Verification items for the finished model (mm, model axes). A direction names the side the tool comes from. Coordinates: 2 decimals unless noted, no trailing zeros. Write each loop counter-clockwise with the first axis right and the second up, starting at its lowest first coordinate (ties: lowest second). Pieces come first, ordered by that corner, then holes. Notation, with made-up numbers: (54.5, -33) - (60.5, -33) arc R34 ccw to (60.5, 1) - close; hole circle Ø4 at (48.25, -30.5). An arc over 180 degrees is marked (long way). Use CSV: the item, a comma, the result in double quotes. Start each with the question number.
```python
from build123d import *

# Parameters (mm, degrees)
F0_R     = 3
F0_R_2   = 2.5
F1_DEPTH = 25


with BuildPart() as f1:
    # F0 (on Top) → F1 (new body)
    with BuildSketch(Plane.XY):
        with BuildLine():
            ThreePointArc((-14.5, 15), (-14.853553, 14.853553), (-15, 14.5))
            Line((-15, 14.5), (-15, 3.15))
            Line((-15, 3.15), (-12.5, 3.15))
            Line((-12.5, 3.15), (-12.5, 5.5))
            Line((-12.5, 5.5), (-6.90098, 5.5))
            ThreePointArc((-6.90098, 5.5), (-5.126404, 3.000613), (-4.5, 0))
            ThreePointArc((-4.5, 0), (-5.126404, -3.000613), (-6.90098, -5.5))
            Line((-6.90098, -5.5), (-12.5, -5.5))
            Line((-12.5, -5.5), (-12.5, -3.15))
            Line((-12.5, -3.15), (-15, -3.15))
            Line((-15, -3.15), (-15, -14.5))
            ThreePointArc((-15, -14.5), (-14.853553, -14.853553), (-14.5, -15))
            Line((-14.5, -15), (-3.15, -15))
            Line((-3.15, -15), (-3.15, -12.5))
            Line((-3.15, -12.5), (-5.5, -12.5))
            Line((-5.5, -12.5), (-5.5, -6.90098))
            ThreePointArc((-5.5, -6.90098), (-3.000613, -5.126404), (0, -4.5))
            ThreePointArc((0, -4.5), (3.000613, -5.126404), (5.5, -6.90098))
            Line((5.5, -6.90098), (5.5, -12.5))
            Line((5.5, -12.5), (3.15, -12.5))
            Line((3.15, -12.5), (3.15, -15))
            Line((3.15, -15), (14.5, -15))
            ThreePointArc((14.5, -15), (14.853553, -14.853553), (15, -14.5))
            Line((15, -14.5), (15, -3.15))
            Line((15, -3.15), (12.5, -3.15))
            Line((12.5, -3.15), (12.5, -5.5))
            Line((12.5, -5.5), (6.90098, -5.5))
            ThreePointArc((6.90098, -5.5), (5.126404, -3.000613), (4.5, 0))
            ThreePointArc((4.5, 0), (5.126404, 3.000613), (6.90098, 5.5))
            Line((6.90098, 5.5), (12.5, 5.5))
            Line((12.5, 5.5), (12.5, 3.15))
            Line((12.5, 3.15), (15, 3.15))
            Line((15, 3.15), (15, 14.5))
            ThreePointArc((15, 14.5), (14.853553, 14.853553), (14.5, 15))
            Line((14.5, 15), (3.15, 15))
            Line((3.15, 15), (3.15, 12.5))
            Line((3.15, 12.5), (5.5, 12.5))
            Line((5.5, 12.5), (5.5, 6.90098))
            ThreePointArc((5.5, 6.90098), (3.000613, 5.126404), (0, 4.5))
            ThreePointArc((0, 4.5), (-3.000613, 5.126404), (-5.5, 6.90098))
            Line((-5.5, 6.90098), (-5.5, 12.5))
            Line((-5.5, 12.5), (-3.15, 12.5))
            Line((-3.15, 12.5), (-3.15, 15))
            Line((-3.15, 15), (-14.5, 15))
        make_face()
        with Locations((-10, -10)):
            Circle(F0_R, mode=Mode.SUBTRACT)
        with Locations((10, -10)):
            Circle(F0_R, mode=Mode.SUBTRACT)
        Circle(F0_R_2, mode=Mode.SUBTRACT)
        with Locations((-10, 10)):
            Circle(F0_R, mode=Mode.SUBTRACT)
        with Locations((10, 10)):
            Circle(F0_R, mode=Mode.SUBTRACT)
    extrude(amount=F1_DEPTH)


solid = f1.part
```
Q1. Gauge pin test, flat end, axial feed: pin 1 (3 mm diameter, centred on x = 0, z = 11, fed in from -Y). Record the tip position at first contact, or that the pin passes through.
Q2. Cross-section at D-D (y = 0.5). Record the cut outline in (x, z), plus the area to 3 significant figures.
Q3. Cross-section at A-A (y = -10). Record the cut outline in (x, z), plus the area to 3 significant figures.
Q4. Scan lines: line 1 along Y through (x, z) = (10, 13.25); line 2 along Y through (x, z) = (-11.5, 5); line 3 along X through (y, z) = (-8, 5.25). Record each from-to range of solid material in increasing order. Write a range as from..to.
Q5. Tool access check on faces 1 (the flat face through (14, 3.15, 12)), 2 (the flat face through (4, -12.5, 12)). Record the directions out of +Z, -Z, +X, -X, +Y, -Y that give a thin tool (end or side, any length) a straight path to the whole face; none if there is none.
Q6. Cross-section at C-C (x = 1.75). Record the cut outline in (y, z).
Q7. Release check for a two-part mould opening along Y. For faces 3 (the flat face through (15, 9, 12)), 4 (the flat face through (-9, -15, 12)), 5 (the flat face through (10, -5.5, 12)), 6 (the flat face through (9, 15, 12)) record: released by +Y, released by -Y, zero draft, split by the parting line, or undercut.
Reply:
1,pin 1,"y = -4.65"
2,outline,"(-4.52, 0) - (-2.45, 0) - (-2.45, 25) - (-4.52, 25) - close; (2.45, 0) - (4.52, 0) - (4.52, 25) - (2.45, 25) - close"
2,area,"103 mm^2"
3,outline,"(-15, 0) - (-13, 0) - (-13, 25) - (-15, 25) - close; (-7, 0) - (-5.5, 0) - (-5.5, 25) - (-7, 25) - close; (5.5, 0) - (7, 0) - (7, 25) - (5.5, 25) - close; (13, 0) - (15, 0) - (15, 25) - (13, 25) - close"
3,area,"175 mm^2"
4,line 1,"-15..-13, -7..-5.5, 5.5..7, 13..15"
4,line 2,"-15..-12.6, -7.4..-5.5, 5.5..7.4, 12.6..15"
4,line 3,"-15..-12.24, -7.76..-5.5, 5.5..7.76, 12.24..15"
5,face 1,"+Z, -Z, +X"
5,face 2,"+Z, -Z"
6,outline,"(-4.71, 0) - (-1.79, 0) - (-1.79, 25) - (-4.71, 25) - close; (1.79, 0) - (4.71, 0) - (4.71, 25) - (1.79, 25) - close"
7,face 3,"zero draft"
7,face 4,"released by -Y"
7,face 5,"undercut"
7,face 6,"released by +Y"
